Can you work these out from the model? Positions are in its coordinate system, mm. Face numbers are marked on the shaded views. Give positions to 0.01 mm unless a question says otherwise; leave off trailing zeros. Order: outer loops, then holes, each group sorted by start corner. A loop starts at its lowest first (then second) coordinate and runs counter-clockwise, first axis right, second up.
Item 1: I'm going to push flat-ended pins straight in: pin 1 Ø1 at (x, y) = (-1, 14) entering from -Z; pin 2 Ø11.5 at (x, y) = (-11, -21.5) entering from -Z. Where does each tip first touch, or does it pass through?
Item 2: I want a section at B-B, the plane y = -18.5. Write out the boundary of the cut face in (x, z), then the cut area to 3 significant figures.
Item 3: I want a section at C-C, the plane z = 1.8. Write out the boundary of the cut face in (x, y), then the cut area to 3 significant figures.
Item 4: If I drill on line 1 along Z through (x, y) = (2.5, -20); line 2 along Z through (x, y) = (-10, -4); line 3 along Y through (x, z) = (-12.5, -0.05), over which ranges is the centre line in solid material (lowest first)?
Item 5: I want a section at A-A, the plane x = -2. Write out the boundary of the cut face in (y, z), then the cut area to 3 significant figures.
Item 6: If we mould it in two halves opening along Y, with no side actions, what happens to the marked faces 1 and 2? For each: +Y half, -Y half, draft (parallel to the pull), parting line (faces both ways), or undercut.
Item 7: I want a section at D-D, the plane y = 7.5. Write out the boundary of the cut face in (x, z).
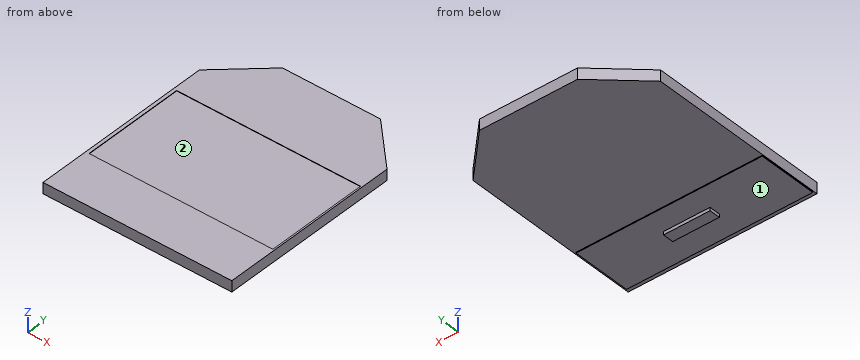
```python
from build123d import *

# Parameters (mm, degrees)
PAD023_DEPTH    = 2.7
SKETCH025_W     = 45.482226
SKETCH025_H     = 25.470864
POCKET004_DEPTH = 0.1
SKETCH026_W     = 11.525024
SKETCH026_H     = 2.6917
PAD024_DEPTH    = 1
SKETCH027_W     = 46.067685
SKETCH027_H     = 14.680909
PAD025_DEPTH    = 0.2


with BuildPart() as part:
    # Sketch024 → Pad023 (new body)
    with BuildSketch(Plane.XY):
        Polygon((-12.752221, 28.783382), (11.516397, 28.783382), (22.453339, 17.81637), (22.453339, -27.300421), (-24.258354, -27.300421), (-24.258354, 18.181068), align=None)
    extrude(amount=PAD023_DEPTH)

    # Sketch025 (on Face8 of Pad023) → Pocket004 (cut)
    with BuildSketch(Plane.XY.offset(2.7)):
        with Locations((-0.682435, -2.157326)):
            Rectangle(SKETCH025_W, SKETCH025_H)
    extrude(amount=-POCKET004_DEPTH, mode=Mode.SUBTRACT)

    # Sketch026 (on Face4 of Pocket004) → Pad024 (join)
    with BuildSketch(Plane(origin=(0, 0, 0), x_dir=(1, 0, 0), z_dir=(0, 0, -1))):
        with Locations((-0.606202, 18.569942)):
            Rectangle(SKETCH026_W, SKETCH026_H)
    extrude(amount=PAD024_DEPTH)

    # Sketch027 (on Face4 of Pad024) → Pad025 (join)
    with BuildSketch(Plane(origin=(0, 0, 0), x_dir=(1, 0, 0), z_dir=(0, 0, -1))):
        with Locations((-1.0373535, 18.9408465)):
            Rectangle(SKETCH027_W, SKETCH027_H)
    extrude(amount=PAD025_DEPTH)


solid = part.part
```
Results list:
1. pin 1: stops at z = 0
1. pin 2: stops at z = -1
2. outline: (-24.26, 0) - (-24.07, 0) - (-24.07, -0.2) - (-6.37, -0.2) - (-6.37, -1) - (5.16, -1) - (5.16, -0.2) - (22, -0.2) - (22, 0) - (22.45, 0) - (22.45, 2.7) - (-24.26, 2.7) - close
2. area: 145 mm2
3. outline: (-24.26, -27.3) - (22.45, -27.3) - (22.45, 17.82) - (11.52, 28.78) - (-12.75, 28.78) - (-24.26, 18.18) - close
3. area: 2,500 mm2
4. line 1: z = -0.2 to 2.7
4. line 2: z = 0 to 2.6
4. line 3: y = -26.28 to -11.6
5. outline: (-27.3, 0) - (-26.28, 0) - (-26.28, -0.2) - (-19.92, -0.2) - (-19.92, -1) - (-17.22, -1) - (-17.22, -0.2) - (-11.6, -0.2) - (-11.6, 0) - (28.78, 0) - (28.78, 2.7) - (10.58, 2.7) - (10.58, 2.6) - (-14.89, 2.6) - (-14.89, 2.7) - (-27.3, 2.7) - close
5. area: 154 mm2
6. face 1: draft
6. face 2: undercut
7. outline: (-24.26, 0) - (22.45, 0) - (22.45, 2.7) - (22.06, 2.7) - (22.06, 2.6) - (-23.42, 2.6) - (-23.42, 2.7) - (-24.26, 2.7) - close
